```python
from build123d import *

# Parameters (mm, degrees)
SKETCH1_W           = 110
SKETCH1_H           = 50
SKETCH1_W_2         = 94
SKETCH1_H_2         = 30
BOSS_EXTRUDE1_DEPTH = 10
FILLET1_R           = 5


with BuildPart() as part:
    # Sketch1 → Boss-Extrude1 (new body)
    with BuildSketch(Plane(origin=(0, 0, 0), x_dir=(1, 0, 0), z_dir=(0, 1, 0))):
        Rectangle(SKETCH1_W, SKETCH1_H)
        Rectangle(SKETCH1_W_2, SKETCH1_H_2, mode=Mode.SUBTRACT)
    extrude(amount=BOSS_EXTRUDE1_DEPTH)

    # Fillet1
    fillet1_edges = [part.edges().sort_by_distance(p)[0] for p in [
        (-47, 5, -15),
        (-47, 5, 15),
        (47, 5, 15),
        (47, 5, -15),
        (-55, 5, 25),
        (-55, 5, -25),
        (55, 5, -25),
        (55, 5, 25),
    ]]
    fillet(fillet1_edges, radius=FILLET1_R)


solid = part.part
```
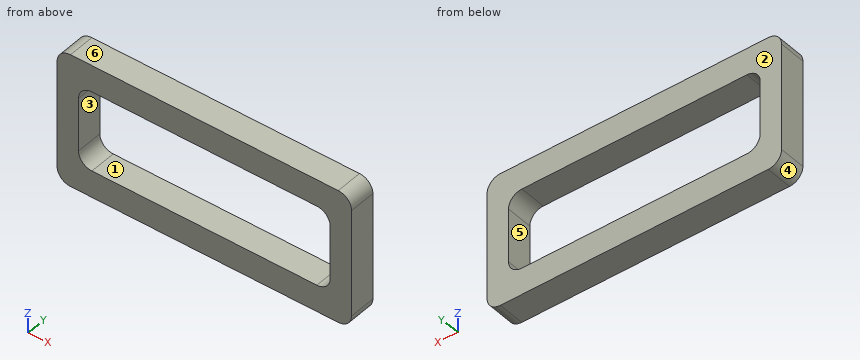
Could you check a few things on this model? Use its own coordinates, in mm. Face numbers are marked on the shaded views. A direction names the side the tool comes from. Round coordinates to 2 decimals unless told otherwise and drop trailing zeros. Loops run counter-clockwise (first coordinate to the right, second up) from the corner with the lowest first, then second, coordinate; pieces in that order, holes last.
Q1. I want a section at C-C (y = 7). Write out the boundary of the cut face in (x, z).
Q2. On a 3-axis mill with a long thin cutter (end or side, diameter ignored), from which of +Z, -Z, +X, -X, +Y, -Y can I reach the whole of each face in a straight line? I mean the marked faces 5 and 6. Say none if no direction works.
Q3. Please list where these lines run through material, in increasing order: L1, parallel to Z at x = 10, y = 2.25; L2, parallel to X at y = 7.25, z = -9.5; L3, parallel to X at y = 4.5, z = 14.
Q4. I want a section at A-A (z = 14). Write out the boundary of the cut face in (x, y).
Q5. Thinking about a two-plate mould opening in X: for the marked faces 1, 2, 3 and 4, which applies, pulls with the +X half, pulls with the -X half, needs draft (parallel to the pull), parting line crosses it, or undercut?
Q6. I want a section at B-B (x = -11). Write out the boundary of the cut face in (y, z).
Answer below:
1. outline: (-55, -20) arc R5 ccw to (-50, -25) - (50, -25) arc R5 ccw to (55, -20) - (55, 20) arc R5 ccw to (50, 25) - (-50, 25) arc R5 ccw to (-55, 20) - close; hole (-47, -10) arc R5 ccw to (-42, -15) - (42, -15) arc R5 ccw to (47, -10) - (47, 10) arc R5 ccw to (42, 15) - (-42, 15) arc R5 ccw to (-47, 10) - close
2. face 5: +Y, -Y
2. face 6: +Z, +X, -X, +Y, -Y
3. L1: z = -25 to -15, 15 to 25
3. L2: x = -55 to -47, 47 to 55
3. L3: x = -55 to -45, 45 to 55
4. outline: (-55, 0) - (-45, 0) - (-45, 10) - (-55, 10) - close; (45, 0) - (55, 0) - (55, 10) - (45, 10) - close
5. face 1: undercut
5. face 2: needs draft
5. face 3: undercut
5. face 4: pulls with the -X half
6. outline: (0, -25) - (10, -25) - (10, -15) - (0, -15) - close; (0, 15) - (10, 15) - (10, 25) - (0, 25) - close
